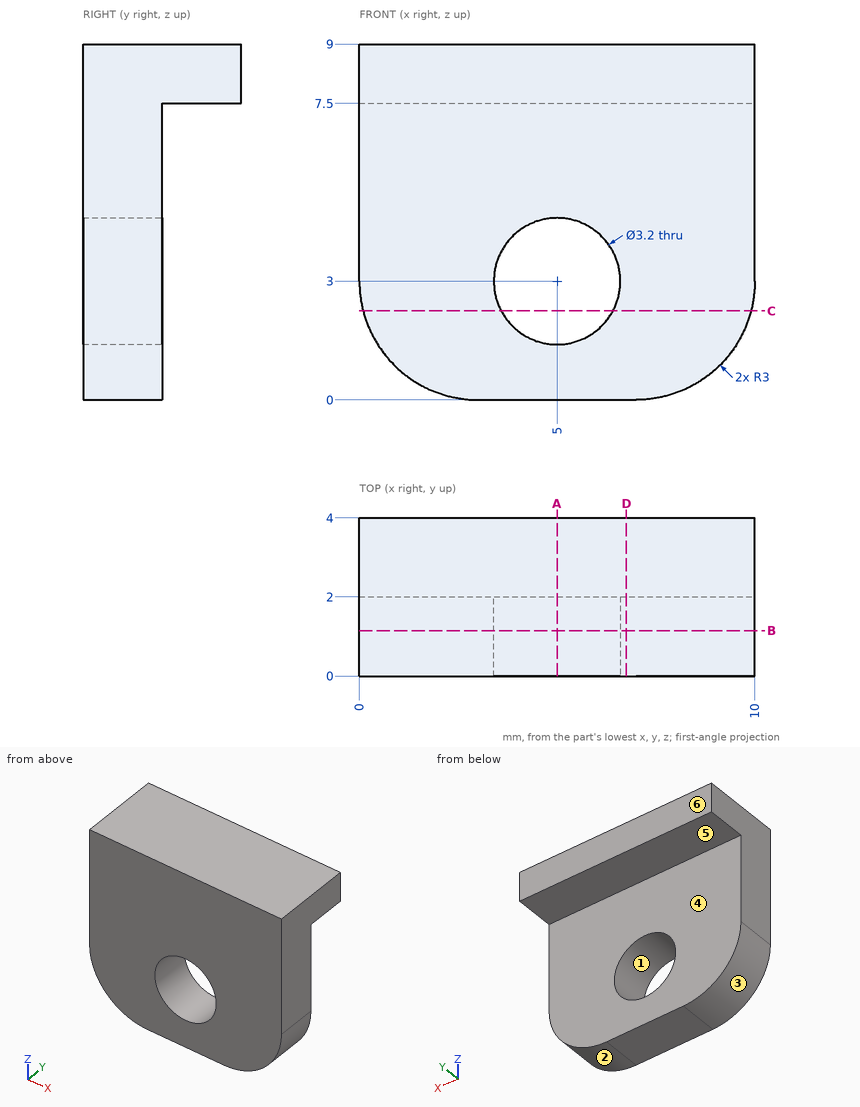
The figure shows three views and two pictorial views of one solid part (mm, origin at its lowest corner). Answer the questions. A direction names the side the tool comes from. Give positions to 0.01 mm unless a question says otherwise; leave off trailing zeros. Write each loop counter-clockwise with the first axis right and the second up, starting at its lowest first coordinate (ties: lowest second). Pieces come first, ordered by that corner, then holes. Notation, with made-up numbers: M 89,54.5 L 104,54.5 A12 ccw 104,66.5 Z; hole C 11,60.5 d11. An arc over 180 degrees is marked long. One line per item, written item: value. Start each with the question number.
(1) Find section A-A (x = 5). Determine the outline of the cut face in (y, z), plus the area to 3 significant figures.
(2) Find section D-D (x = 6.75). Determine the outline of the cut face in (y, z).
(3) Find section B-B (y = 1.15). Determine the outline of the cut face in (x, z).
(4) Flat-ended cylindrical pins translate along their axes: pin 1 Ø2.5 at (x, z) = (5, 3) entering from +Y; pin 2 Ø1 at (x, y) = (5.5, 3) entering from -Z. Find the tip coordinate at first contact, or state that the pin passes through.
(5) Find the intervals of material crossed by line 1 (Z direction, x = 5, y = 1.15); line 2 (Z direction, x = 7.5, y = 3.85); line 3 (Y direction, x = 6.5, z = 6.5), in increasing order.
(6) Find section C-C (z = 2.25). Determine the outline of the cut face in (x, y), plus the area to 3 significant figures.
(7) A tool of negligible diameter and unlimited length cuts with its end or side. For the marked faces 5 and 6, from which of +Z, -Z, +X, -X, +Y, -Y can it reach the whole face along a straight path? Write none if from no direction.
(8) Determine the mould class of the marked faces 1, 2, 3 and 4 for opening direction X: pulls with the +X half, pulls with the -X half, needs draft (parallel to the pull), parting line crosses it, or undercut.
Results below:
1. outline: M 0,0 L 2,0 L 2,1.4 L 0,1.4 Z; M 0,4.6 L 2,4.6 L 2,7.5 L 4,7.5 L 4,9 L 0,9 Z
1. area: 14.6 mm^2
2. outline: M 0,0 L 2,0 L 2,7.5 L 4,7.5 L 4,9 L 0,9 Z
3. outline: M 0,3 A3 ccw 3,0 L 7,0 A3 ccw 10,3 L 10,9 L 0,9 Z; hole C 5,3 d3.2
4. pin 1: passes through
4. pin 2: stops at z = 7.5
5. line 1: z = 0 to 1.4, 4.6 to 9
5. line 2: z = 7.5 to 9
5. line 3: y = 0 to 2
6. outline: M 0.1,0 L 3.59,0 L 3.59,2 L 0.1,2 Z; M 6.41,0 L 9.9,0 L 9.9,2 L 6.41,2 Z
6. area: 14.0 mm^2
7. face 5: -Z, +X, -X, +Y
7. face 6: +Z, -Z, +X, -X, +Y
8. face 1: undercut
8. face 2: pulls with the +X half
8. face 3: pulls with the -X half
8. face 4: needs draft
